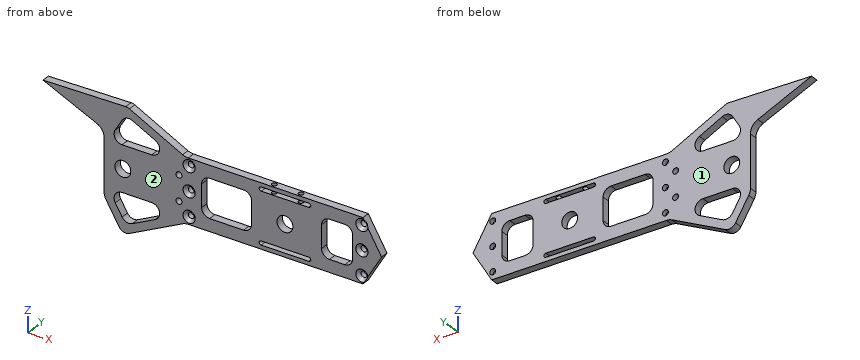
```python
from build123d import *

# Parameters (mm, degrees)
CROQUIS1_R              = 6.35
SALIENTE_EXTRUIR1_DEPTH = 6.35
REDONDEO1_R             = 10
CORTAR_EXTRUIR2_DEPTH   = 225.405229946
CORTAR_EXTRUIR3_DEPTH   = 225.405229946
CROQUIS7_R              = 2.38125
CORTAR_EXTRUIR4_DEPTH   = 225.405229946
CROQUIS8_R              = 2.38125
CORTAR_EXTRUIR5_DEPTH   = 225.405229946
CROQUIS9_R              = 2
CORTAR_EXTRUIR6_DEPTH   = 15
CHAFL_N1_SIZE           = 2.5


with BuildPart() as part:
    # Croquis1 → Saliente-Extruir1 (new body)
    with BuildSketch(Plane(origin=(0, 0, 0), x_dir=(1, 0, 0), z_dir=(0, 1, 0))):
        with BuildLine():
            Line((37.5, -25.4), (52.5, 0))
            Line((52.5, 0), (37.5, 25.4))
            Line((37.5, 25.4), (-105, 25.4))
            Line((-105, 25.4), (-149.746813481, 47.731727951))
            ThreePointArc((-149.746813481, 47.731727951), (-154.357530471, 48.146831931), (-158.024774803, 45.321528145))
            Line((-158.024774803, 45.321528145), (-170, 25.4))
            Line((-170, 25.4), (-170, -25.4))
            Line((-170, -25.4), (-219.03156103, -47.147007635))
            Line((-219.03156103, -47.147007635), (-152.702210171, -48.398869348))
            ThreePointArc((-152.702210171, -48.398869348), (-151.184140049, -48.244143221), (-149.746813481, -47.731727951))
            Line((-149.746813481, -47.731727951), (-105, -25.4))
            Line((-105, -25.4), (37.5, -25.4))
        make_face()
        with Locations(Location((-155, 0, 0), (0, 0, 270))):
            Circle(CROQUIS1_R, mode=Mode.SUBTRACT)
        with Locations(Location((-25, 0, 0), (0, 0, 270))):
            Circle(CROQUIS1_R, mode=Mode.SUBTRACT)
        with BuildLine():
            Line((-129.045100716, 30.303281185), (-147.329198773, 39.428299747))
            ThreePointArc((-147.329198773, 39.428299747), (-151.939915763, 39.843403727), (-155.607160095, 37.018099941))
            Line((-155.607160095, 37.018099941), (-161.092389512, 27.893081378))
            ThreePointArc((-161.092389512, 27.893081378), (-161.177056347, 21.495189828), (-155.65, 18.271553233))
            Line((-155.65, 18.271553233), (-131.880672526, 18.271553233))
            ThreePointArc((-131.880672526, 18.271553233), (-125.699998109, 23.164925706), (-129.045100716, 30.303281185))
        make_face(mode=Mode.SUBTRACT)
        with BuildLine():
            Line((-129.045100716, -30.303281185), (-147.329198773, -39.428299747))
            ThreePointArc((-147.329198773, -39.428299747), (-151.939915763, -39.843403727), (-155.607160095, -37.018099941))
            Line((-155.607160095, -37.018099941), (-161.092389512, -27.893081378))
            ThreePointArc((-161.092389512, -27.893081378), (-161.177056347, -21.495189828), (-155.65, -18.271553233))
            Line((-155.65, -18.271553233), (-131.880672526, -18.271553233))
            ThreePointArc((-131.880672526, -18.271553233), (-125.699998109, -23.164925706), (-129.045100716, -30.303281185))
        make_face(mode=Mode.SUBTRACT)
    extrude(amount=SALIENTE_EXTRUIR1_DEPTH)

    # Redondeo1
    redondeo1_edges = [part.edges().sort_by_distance(p)[0] for p in [
        (-105, 3.175, 25.4),
        (-170, 3.175, 25.4),
        (-170, 3.175, -25.4),
        (-105, 3.175, -25.4),
    ]]
    fillet(redondeo1_edges, radius=REDONDEO1_R)

    # Croquis5 → Cortar-Extruir2 (cut, through all)
    with BuildSketch(Plane.XZ):
        with BuildLine():
            Line((-44.125, 22.225), (-5.875, 22.225))
            ThreePointArc((-5.875, 22.225), (-4.2875, 20.6375), (-5.875, 19.05))
            Line((-5.875, 19.05), (-44.125, 19.05))
            ThreePointArc((-44.125, 19.05), (-45.7125, 20.6375), (-44.125, 22.225))
        make_face()
        with BuildLine():
            Line((-5.875, -19.05), (-44.125, -19.05))
            ThreePointArc((-44.125, -19.05), (-45.7125, -20.6375), (-44.125, -22.225))
            Line((-44.125, -22.225), (-5.875, -22.225))
            ThreePointArc((-5.875, -22.225), (-4.2875, -20.6375), (-5.875, -19.05))
        make_face()
    extrude(amount=-CORTAR_EXTRUIR2_DEPTH, mode=Mode.SUBTRACT)

    # Croquis6 → Cortar-Extruir3 (cut, through all)
    with BuildSketch(Plane.XZ):
        with BuildLine():
            Line((-85.475, 15.4), (-58.175, 15.4))
            ThreePointArc((-58.175, 15.4), (-53.684871939, 13.540128061), (-51.825, 9.05))
            Line((-51.825, 9.05), (-51.825, -9.05))
            ThreePointArc((-51.825, -9.05), (-53.684871939, -13.540128061), (-58.175, -15.4))
            Line((-58.175, -15.4), (-85.475, -15.4))
            ThreePointArc((-85.475, -15.4), (-89.965128061, -13.540128061), (-91.825, -9.05))
            Line((-91.825, -9.05), (-91.825, 9.05))
            ThreePointArc((-91.825, 9.05), (-89.965128061, 13.540128061), (-85.475, 15.4))
        make_face()
        with BuildLine():
            Line((10.675, 15.4), (22.975, 15.4))
            ThreePointArc((22.975, 15.4), (27.465128061, 13.540128061), (29.325, 9.05))
            Line((29.325, 9.05), (29.325, -9.05))
            ThreePointArc((29.325, -9.05), (27.465128061, -13.540128061), (22.975, -15.4))
            Line((22.975, -15.4), (10.675, -15.4))
            ThreePointArc((10.675, -15.4), (6.184871939, -13.540128061), (4.325, -9.05))
            Line((4.325, -9.05), (4.325, 9.05))
            ThreePointArc((4.325, 9.05), (6.184871939, 13.540128061), (10.675, 15.4))
        make_face()
    extrude(amount=-CORTAR_EXTRUIR3_DEPTH, mode=Mode.SUBTRACT)

    # Croquis7 → Cortar-Extruir4 (cut, through all)
    with BuildSketch(Plane.XZ):
        with Locations(Location((-101.825, 0, 0), (0, 0, 270))):
            Circle(CROQUIS7_R)
        with Locations(Location((-101.825, 19.4, 0), (0, 0, 270))):
            Circle(CROQUIS7_R)
        with Locations(Location((-101.825, -19.4, 0), (0, 0, 270))):
            Circle(CROQUIS7_R)
        with Locations(Location((36.681745283, -19.4, 0), (0, 0, 90))):
            Circle(CROQUIS7_R)
        with Locations(Location((36.681745283, 19.4, 0), (0, 0, 90))):
            Circle(CROQUIS7_R)
        with Locations(Location((36.681745283, 0, 0), (0, 0, 90))):
            Circle(CROQUIS7_R)
    extrude(amount=-CORTAR_EXTRUIR4_DEPTH, mode=Mode.SUBTRACT)

    # Croquis8 → Cortar-Extruir5 (cut, through all)
    with BuildSketch(Plane.XZ):
        with Locations(Location((-110, -10, 0), (0, 0, 270))):
            Circle(CROQUIS8_R)
        with Locations(Location((-110, 10, 0), (0, 0, 270))):
            Circle(CROQUIS8_R)
    extrude(amount=-CORTAR_EXTRUIR5_DEPTH, mode=Mode.SUBTRACT)

    # Croquis9 → Cortar-Extruir6 (cut)
    with BuildSketch(Plane.XY.offset(25.4)):
        with Locations((-14.2875, 3.175)):
            Circle(CROQUIS9_R)
        with Locations((-35.7125, 3.175)):
            Circle(CROQUIS9_R)
    extrude(amount=-CORTAR_EXTRUIR6_DEPTH, mode=Mode.SUBTRACT)

    # Chaflán1
    # the kernel refuses this chamfer: 2.5 mm, written as the material it takes off along each edge
    with BuildSketch(Plane(origin=(-101.825, 0, 19.4), x_dir=(0, 0, -1), z_dir=(-1, 0, 0))) as chafl_n1_piece_1:
        Polygon((2.38125 + CHAFL_N1_SIZE, 0), (2.38125, -CHAFL_N1_SIZE), (2.38125, 0), align=None)
    revolve(axis=Axis((-101.825, 0, 19.4), (0, -1, 0)), mode=Mode.SUBTRACT)
    with BuildSketch(Plane(origin=(-101.825, 0, -19.4), x_dir=(0, 0, -1), z_dir=(-1, 0, 0))) as chafl_n1_piece_2:
        Polygon((2.38125 + CHAFL_N1_SIZE, 0), (2.38125, -CHAFL_N1_SIZE), (2.38125, 0), align=None)
    revolve(axis=Axis((-101.825, 0, -19.4), (0, -1, 0)), mode=Mode.SUBTRACT)
    with BuildSketch(Plane(origin=(36.681745283, 0, -19.4), x_dir=(0, 0, 1), z_dir=(1, 0, 0))) as chafl_n1_piece_3:
        Polygon((2.38125 + CHAFL_N1_SIZE, 0), (2.38125, -CHAFL_N1_SIZE), (2.38125, 0), align=None)
    revolve(axis=Axis((36.681745283, 0, -19.4), (0, -1, 0)), mode=Mode.SUBTRACT)
    with BuildSketch(Plane(origin=(36.681745283, 0, 19.4), x_dir=(0, 0, 1), z_dir=(1, 0, 0))) as chafl_n1_piece_4:
        Polygon((2.38125 + CHAFL_N1_SIZE, 0), (2.38125, -CHAFL_N1_SIZE), (2.38125, 0), align=None)
    revolve(axis=Axis((36.681745283, 0, 19.4), (0, -1, 0)), mode=Mode.SUBTRACT)
    with BuildSketch(Plane(origin=(36.681745283, 0, 0), x_dir=(0, 0, 1), z_dir=(1, 0, 0))) as chafl_n1_piece_5:
        Polygon((2.38125 + CHAFL_N1_SIZE, 0), (2.38125, -CHAFL_N1_SIZE), (2.38125, 0), align=None)
    revolve(axis=Axis((36.681745283, 0, 0), (0, -1, 0)), mode=Mode.SUBTRACT)
    with BuildSketch(Plane(origin=(-101.825, 0, 0), x_dir=(0, 0, -1), z_dir=(-1, 0, 0))) as chafl_n1_piece_6:
        Polygon((2.38125 + CHAFL_N1_SIZE, 0), (2.38125, -CHAFL_N1_SIZE), (2.38125, 0), align=None)
    revolve(axis=Axis((-101.825, 0, 0), (0, -1, 0)), mode=Mode.SUBTRACT)


solid = part.part
```
For this review, take the finished solid that the model builds, in its own axes (mm). Face numbers are marked on the shaded views. Round coordinates to 2 decimals unless told otherwise and drop trailing zeros. Order: outer loops, then holes, each group sorted by start corner. A loop starts at its lowest first (then second) coordinate and runs counter-clockwise, first axis right, second up. Notation, with made-up numbers: (57, 30) -> (77, 30) arc R19 ccw to (77, 52) -> close; hole circle Ø6 at (11, -33). An arc over 180 degrees is marked (long way). Use a Markdown table: item, result.
Item 1: Take a section at A-A (x = -40.5). State the section outline as (y, z) points (3 decimals), plus the area to 3 significant figures.
Resolved:
| item | result |
|---|---|
| outline | (0, -25.4) -> (6.35, -25.4) -> (6.35, -22.225) -> (0, -22.225) -> close; (0, -19.05) -> (6.35, -19.05) -> (6.35, 19.05) -> (0, 19.05) -> close; (0, 22.225) -> (6.35, 22.225) -> (6.35, 25.4) -> (0, 25.4) -> close |
| area | 282 mm² |
Item 2: Take a section at C-C (x = -193.5). State the section outline as (y, z) points.
Resolved:
| item | result |
|---|---|
| outline | (0, 35.82) -> (6.35, 35.82) -> (6.35, 47.63) -> (0, 47.63) -> close |
Item 3: Draft analysis for pull direction Y (two halves, no side actions). For the marked faces 1 and 2, state which applies: +Y half, -Y half, draft (parallel to the pull), parting line (faces both ways), or undercut.
Resolved:
| item | result |
|---|---|
| face 1 | +Y half |
| face 2 | -Y half |
Item 4: For line 1 along Z through (x, y) = (-9, 2.25) (3 decimals); line 2 along Z through (x, y) = (-135, 1.25); line 3 along Z through (x, y) = (-80, 3), list the stretches that pass through material, from the lowest coordinate up. Write a range as [from, to].
Resolved:
| item | result |
|---|---|
| line 1 | z = [-25.4, -22.225], [-19.05, 19.05], [22.225, 25.4] |
| line 2 | z = [-40.37, -33.28], [-18.27, 18.27], [33.28, 40.37] |
| line 3 | z = [-25.4, -15.4], [15.4, 25.4] |
Item 5: Take a section at B-B (x = -110). State the section outline as (y, z) points, plus the area to 3 significant figures.
Resolved:
| item | result |
|---|---|
| outline | (0, -27.9) -> (6.35, -27.9) -> (6.35, -12.38) -> (0, -12.38) -> close; (0, -7.62) -> (6.35, -7.62) -> (6.35, 7.62) -> (0, 7.62) -> close; (0, 12.38) -> (6.35, 12.38) -> (6.35, 27.9) -> (0, 27.9) -> close |
| area | 294 mm² |
Item 6: For pin 1 (6 mm diameter, centred on x = -101.825, z = -19.4, fed in from +Y); pin 2 (1 mm diameter, centred on x = -156, y = 3.5, fed in from +Z); pin 3 (4 mm diameter, centred on x = 36.68, z = 19.4, fed in from -Y); pin 4 (2 mm diameter, centred on x = -124.5, y = 1.5, fed in from -Z), all flat-tipped, find the tip position at first contact; note any pin that passes through.
Resolved:
| item | result |
|---|---|
| pin 1 | stops at y = 6.35 |
| pin 2 | stops at z = 48.35 |
| pin 3 | passes through |
| pin 4 | stops at z = -35.63 |
